Autodesk Inventor part; units mm, degrees
ref_plane "YZ Plane" through (0, 0, 0) normal (1, 0, 0) x (0, 1, 0)
ref_plane "XZ Plane" through (0, 0, 0) normal (0, 1, 0) x (-1, 0, 0)
ref_plane "XY Plane" through (0, 0, 0) normal (0, 0, 1) x (1, 0, 0)
sketch "スケッチ1" plane through (0, 0, 0) normal (0, 0, 1) x (1, 0, 0)
  line L0 (0, 0) -> (0, 3)
  line L1 (0, 3) -> (0.2, 3)
  line L2 (0.2, 3) -> (1.7, 1.5)
  line L3 (1.7, 1.5) -> (9.7, 1.5)
  line L4 (9.7, 1.5) -> (9.7, 0)
  line L5 (0, 0) -> (9.7, 0)
  dimension "d0" = 45
  dimension "d1" = 3
  dimension "d2" = 1.7
  dimension "d3" = 1.5
  dimension "d4" = 8
revolve "回転1" add sketch "スケッチ1" angle 360 about axis through (0, 0, 0) along (1, 0, 0)
thread "ねじ1"
sketch "スケッチ2" plane through (0, 0, 0) normal (-1, 0, 0) x (0, 0, 1)
  line L0 (0.5774, 1) -> (1.1547, 0)
  line L1 (1.1547, 0) -> (0.5774, -1)
  line L2 (0.5774, -1) -> (-0.5774, -1)
  line L3 (-0.5774, -1) -> (-1.1547, 0)
  line L4 (-1.1547, 0) -> (-0.5774, 1)
  line L5 (-0.5774, 1) -> (0.5774, 1)
  circle A0 centre (0, 0) radius 1.1547
  point P0 (0, 0)
  point P1 (0, 0)
  dimension "d8" = 2
extrude "押し出し1" cut sketch "スケッチ2" against normal blind 1.2 contours L0 L1 L2 L3 L4 L5
chamfer "面取り1" distance 0.05 angle 45 6 edges at (0, -0.5, -0.866) (0, 0.5, -0.866) (0, 1, 0) (0, 0.5, 0.866) (0, -1, 0) (0, -0.5, 0.866)
chamfer "面取り2" distance 0.15 angle 45 1 edges at (9.7, -1.5, 0)
properties part number "ネジ皿M3L8" material "鋼、高強度、低合金"
Geometry check sheet. Reference: the model listing, model coordinates, mm. A direction names the side the tool comes from. Round coordinates to 2 decimals unless told otherwise and drop trailing zeros. Loops run counter-clockwise (first coordinate to the right, second up) from the corner with the lowest first, then second, coordinate; pieces in that order, holes last.
Item 1: Thickness scan on line 1 (Y direction, x = 2, z = 0.6); line 2 (Z direction, x = 2.5, y = -0.7); line 3 (Y direction, x = 3.25, z = 0.85). Record the ranges inside material, lowest first.
Item 2: Access from +Z, -Z, +X, -X, +Y, -Y to the whole of each face (thin tool, end or side, straight path). Record for faces 4 (the flat face through (0.62, -0.51, -0.86)), 5 (the flat face through (9.7, 0, 0)).
Item 3: Mould release check, pull along Y, two halves, no side actions. Record for faces 1 (the cylindrical face through (5.68, -1.5, 0.07)), 2 (the flat face through (0.62, 0.49, -0.87)), 3 (the flat face through (0, 1.3, 0)): pulls with the +Y half, pulls with the -Y half, needs draft (parallel to the pull), parting line crosses it, or undercut.
Item 4: Gauge pin test, flat ends, axial feed: pin 1 (2 mm diameter, centred on x = 8, z = -1.5, fed in from -Y); pin 2 (2 mm diameter, centred on x = 6.5, y = -2, fed in from -Z); pin 3 (0.9 mm diameter, centred on x = 0.5, z = -0.5, fed in from +Y). Record the tip position at first contact, or that the pin passes through.
Item 5: Cross-section at A-A on z = 0. Record the boundary of the cut face in (x, y), then the cut area to 3 significant figures.
Item 6: Cross-section at B-B on x = 5.25. Record the boundary of the cut face in (y, z), then the cut area to 3 significant figures.
Answer sheet:
1. line 1: y = -1.37 to 1.37
1. line 2: z = -1.33 to 1.33
1. line 3: y = -1.24 to 1.24
2. face 4: -X
2. face 5: +Z, -Z, +X, +Y, -Y
3. face 1: parting line crosses it
3. face 2: undercut
3. face 3: needs draft
4. pin 1: stops at y = -1.41
4. pin 2: stops at z = -1.12
4. pin 3: stops at y = 3
5. outline: (0, -3) - (0.2, -3) - (1.7, -1.5) - (9.55, -1.5) - (9.7, -1.35) - (9.7, 1.35) - (9.55, 1.5) - (1.7, 1.5) - (0.2, 3) - (0, 3) - (0, 1.05) - (0.05, 1) - (1.2, 1) - (1.2, -1) - (0.05, -1) - (0, -1.05) - close
5. area: 29.5 mm2
6. outline: circle Ø3 at (0, 0)
6. area: 7.07 mm2
